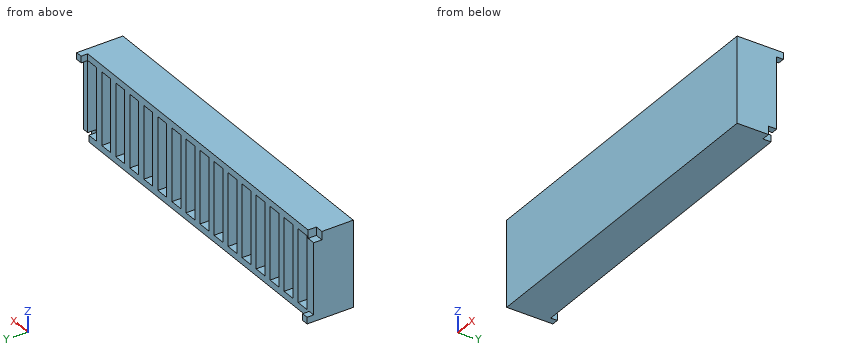
```python
from build123d import *

# Parameters (mm, degrees)
SKETCH1_W           = 104
SKETCH1_H           = 26
BOSS_EXTRUDE1_DEPTH = 12
SKETCH2_W           = 4
SKETCH2_H           = 22
CUT_EXTRUDE1_DEPTH  = 11
SKETCH3_W           = 2
SKETCH3_H           = 2
BOSS_EXTRUDE2_DEPTH = 2
SKETCH4_W           = 2.5
SKETCH4_H           = 2.5
CUT_EXTRUDE2_DEPTH  = 2.5


with BuildPart() as part:
    # Sketch1 → Boss-Extrude1 (new body)
    with BuildSketch(Plane(origin=(0, 0, 0), x_dir=(1, 0, 0), z_dir=(0, 1, 0))):
        Rectangle(SKETCH1_W, SKETCH1_H)
    extrude(amount=BOSS_EXTRUDE1_DEPTH)

    # Sketch2 → Cut-Extrude1 (cut)
    with BuildSketch(Plane(origin=(0, 12, 0), x_dir=(1, 0, 0), z_dir=(0, 1, 0))):
        with Locations((-47, 0)):
            Rectangle(SKETCH2_W, SKETCH2_H)
        with Locations((-40.666666667, 0)):
            Rectangle(SKETCH2_W, SKETCH2_H)
        with Locations((-34.333333333, 0)):
            Rectangle(SKETCH2_W, SKETCH2_H)
        with Locations((-28, 0)):
            Rectangle(SKETCH2_W, SKETCH2_H)
        with Locations((-21.666666667, 0)):
            Rectangle(SKETCH2_W, SKETCH2_H)
        with Locations((-15.333333333, 0)):
            Rectangle(SKETCH2_W, SKETCH2_H)
        with Locations((-9, 0)):
            Rectangle(SKETCH2_W, SKETCH2_H)
        with Locations((-2.666666667, 0)):
            Rectangle(SKETCH2_W, SKETCH2_H)
        with Locations((3.666666667, 0)):
            Rectangle(SKETCH2_W, SKETCH2_H)
        with Locations((10, 0)):
            Rectangle(SKETCH2_W, SKETCH2_H)
        with Locations((16.333333333, 0)):
            Rectangle(SKETCH2_W, SKETCH2_H)
        with Locations((22.666666667, 0)):
            Rectangle(SKETCH2_W, SKETCH2_H)
        with Locations((29, 0)):
            Rectangle(SKETCH2_W, SKETCH2_H)
        with Locations((35.333333333, 0)):
            Rectangle(SKETCH2_W, SKETCH2_H)
        with Locations((41.666666667, 0)):
            Rectangle(SKETCH2_W, SKETCH2_H)
        with Locations((48, 0)):
            Rectangle(SKETCH2_W, SKETCH2_H)
    extrude(amount=-CUT_EXTRUDE1_DEPTH, mode=Mode.SUBTRACT)

    # Sketch3 → Boss-Extrude2 (add)
    with BuildSketch(Plane(origin=(0, 12, 0), x_dir=(1, 0, 0), z_dir=(0, 1, 0))):
        with Locations((-51, 12)):
            Rectangle(SKETCH3_W, SKETCH3_H)
        with Locations((51, -12)):
            Rectangle(SKETCH3_W, SKETCH3_H)
    extrude(amount=BOSS_EXTRUDE2_DEPTH)

    # Sketch4 → Cut-Extrude2 (cut)
    with BuildSketch(Plane(origin=(0, 12, 0), x_dir=(1, 0, 0), z_dir=(0, 1, 0))):
        with Locations((-50.75, -11.75)):
            Rectangle(SKETCH4_W, SKETCH4_H)
        with Locations((50.75, 11.75)):
            Rectangle(SKETCH4_W, SKETCH4_H)
    extrude(amount=-CUT_EXTRUDE2_DEPTH, mode=Mode.SUBTRACT)


solid = part.part
```
Work out the finished part from the listing and answer in its coordinate system (mm). Round coordinates to 2 decimals unless told otherwise and drop trailing zeros. Write each loop counter-clockwise with the first axis right and the second up, starting at its lowest first coordinate (ties: lowest second). Pieces come first, ordered by that corner, then holes. Notation, with made-up numbers: (0, 19.25) -> (52, 19.25) arc R10 ccw to (52, 33.25) -> close; hole circle Ø9 at (39, 34.5). An arc over 180 degrees is marked (long way). Write each question's results on one line, items separated by ' | '.
1) Consider line 1 along Z through (x, y) = (-10, 1.5); line 2 along Y through (x, z) = (-26.5, -8); line 3 along X through (y, z) = (9.75, -11.5). Determine where each line is inside the solid, lowest interval first. Write a range as [from, to].
Findings:
line 1: z = [-13, -11], [11, 13] | line 2: y = [0, 1] | line 3: x = [-52, 49.5]
2) The part is cut by section B-B (y = 6.25). State how many separate pieces and enclosed holes the cut face has, and give its area (3 significant figures).
Findings:
separate pieces: 1 | enclosed holes: 16 | area: 1,300 mm²
3) Flat-ended cylindrical pins translate along their axes: pin 1 (1 mm diameter, centred on x = 15, z = -3, fed in from +Y); pin 2 (1.6 mm diameter, centred on y = 13, z = 12, fed in from -X); pin 3 (4.5 mm diameter, centred on x = -34, z = -1.5, fed in from +Y). Find the tip coordinate at first contact, or state that the pin passes through.
Findings:
pin 1: stops at y = 1 | pin 2: stops at x = 50 | pin 3: stops at y = 12
4) The part is cut by section A-A (x = 10.5). Write down the section's boundary in (y, z), and give its area (3 significant figures).
Findings:
outline: (0, -13) -> (12, -13) -> (12, -11) -> (1, -11) -> (1, 11) -> (12, 11) -> (12, 13) -> (0, 13) -> close | area: 70.0 mm²
5) The part is cut by section C-C (x = 38.5). Write down the section's boundary in (y, z).
Findings:
outline: (0, -13) -> (12, -13) -> (12, 13) -> (0, 13) -> close
